Could you check a few things on this model? Use its own coordinates, in mm. Face numbers are marked on the shaded views. A direction names the side the tool comes from. Round coordinates to 2 decimals unless told otherwise and drop trailing zeros. Write each loop counter-clockwise with the first axis right and the second up, starting at its lowest first coordinate (ties: lowest second). Pieces come first, ordered by that corner, then holes. Notation, with made-up numbers: (21.5, -30) -> (79.5, -30) arc R11 cw to (79.5, -25) -> close; hole circle Ø8 at (10, 88.5). An arc over 180 degrees is marked (long way). Answer in a Markdown table with one row per item.
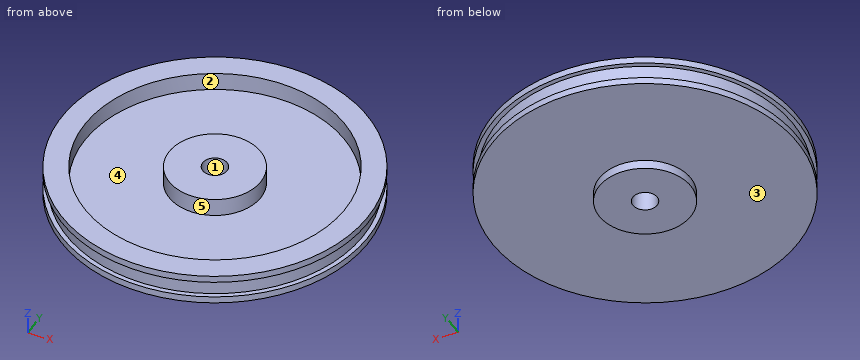
from build123d import *

# Parameters (mm, degrees)
SKETCH_1_R          = 100
EXTRUDE_1_DEPTH     = 20
SKETCH_2_R          = 8
CUT_EXTRUDE_1_DEPTH = 20
SKETCH_3_R          = 85
SKETCH_3_R_2        = 30
CUT_EXTRUDE_2_DEPTH = 12
SKETCH_5_W          = 3
SKETCH_5_H          = 11
SKETCH_8_R          = 30
EXTRUDE_2_DEPTH     = 6
CUT_EXTRUDE_START   = -52
SKETCH_9_R          = 8
CUT_EXTRUDE_4_DEPTH = 52


with BuildPart() as part:
    # 草图1 → 凸台-拉伸1 (new body)
    with BuildSketch(Plane.XY):
        Circle(SKETCH_1_R)
    extrude(amount=EXTRUDE_1_DEPTH)

    # 草图2 → 切除-拉伸1 (cut)
    with BuildSketch(Plane.XY.offset(20)):
        Circle(SKETCH_2_R)
    extrude(amount=-CUT_EXTRUDE_1_DEPTH, mode=Mode.SUBTRACT)

    # 草图3 → 切除-拉伸2 (cut)
    with BuildSketch(Plane.XY.offset(20)):
        Circle(SKETCH_3_R)
        Circle(SKETCH_3_R_2, mode=Mode.SUBTRACT)
    extrude(amount=-CUT_EXTRUDE_2_DEPTH, mode=Mode.SUBTRACT)

    # 草图5 → 切除-旋转2 (revolve, cut)
    with BuildSketch(Plane(origin=(0, 0, 0), x_dir=(1, 0, 0), z_dir=(0, 1, 0)), mode=Mode.PRIVATE) as cut_revolve_2_sk:
        with Locations((98.5, -10)):
            Rectangle(SKETCH_5_W, SKETCH_5_H)
    revolve(cut_revolve_2_sk.sketch.rotate(Axis((0, 0, -40.303548102), (0, 0, 1)), 180), axis=Axis((0, 0, -40.303548102), (0, 0, 1)), mode=Mode.SUBTRACT)

    # 草图8 → 凸台-拉伸2 (add)
    with BuildSketch(Plane(origin=(0, 0, 0), x_dir=(-1, 0, 0), z_dir=(0, 0, -1))):
        with Locations(Location((0, 0, 0), (0, 0, 180))):
            Circle(SKETCH_8_R)
    extrude(amount=EXTRUDE_2_DEPTH)

    # 草图9 → 切除-拉伸4 (cut)
    with BuildSketch(Plane(origin=(0, 0, -6), x_dir=(-1, 0, 0), z_dir=(0, 0, -1)).offset(CUT_EXTRUDE_START)):
        with Locations(Location((0, 0, 0), (0, 0, 180))):
            Circle(SKETCH_9_R)
    extrude(amount=CUT_EXTRUDE_4_DEPTH, mode=Mode.SUBTRACT)


solid = part.part
1) Imagine slicing it at C-C, the plane y = -50.5. Please give me the cut outline in (x, z).
Findings:
| item | result |
|---|---|
| outline | (-86.31, 0) -> (86.31, 0) -> (86.31, 4.5) -> (82.82, 4.5) -> (82.82, 15.5) -> (86.31, 15.5) -> (86.31, 20) -> (68.37, 20) -> (68.37, 8) -> (-68.37, 8) -> (-68.37, 20) -> (-86.31, 20) -> (-86.31, 15.5) -> (-82.82, 15.5) -> (-82.82, 4.5) -> (-86.31, 4.5) -> close |
2) For pin 1 (1 mm diameter, centred on x = 2, z = 3, fed in from -Y); pin 2 (2 mm diameter, centred on x = -9, z = 15.5, fed in from +Y); pin 3 (3 mm diameter, centred on x = 4.5, y = 63.5, fed in from -Z), each with a flat end and sliding along its axis, tell me the tip position at first contact or that it passes through.
Findings:
| item | result |
|---|---|
| pin 1 | stops at y = -99.99 |
| pin 2 | stops at y = 99.68 |
| pin 3 | stops at z = 0 |
3) Imagine slicing it at D-D, the plane x = -55. Please give me the cut outline in (y, z), plus the area to 3 significant figures.
Findings:
| item | result |
|---|---|
| outline | (-83.52, 0) -> (83.52, 0) -> (83.52, 4.5) -> (79.9, 4.5) -> (79.9, 15.5) -> (83.52, 15.5) -> (83.52, 20) -> (64.81, 20) -> (64.81, 8) -> (-64.81, 8) -> (-64.81, 20) -> (-83.52, 20) -> (-83.52, 15.5) -> (-79.9, 15.5) -> (-79.9, 4.5) -> (-83.52, 4.5) -> close |
| area | 1,710 mm^2 |
4) Please list where these lines run through material, in increasing order: line 1 (Y direction, x = 0, z = 14.5); line 2 (Y direction, x = 0, z = 2.25); line 3 (Y direction, x = -16, z = 12.5).
Findings:
| item | result |
|---|---|
| line 1 | y = -97 to -85, -30 to -8, 8 to 30, 85 to 97 |
| line 2 | y = -100 to -8, 8 to 100 |
| line 3 | y = -95.67 to -83.48, -25.38 to 25.38, 83.48 to 95.67 |
5) Imagine slicing it at A-A, the plane y = 0. Please give me the cut outline in (x, z), plus the area to 3 significant figures.
Findings:
| item | result |
|---|---|
| outline | (-100, 0) -> (-30, 0) -> (-30, -6) -> (-8, -6) -> (-8, 20) -> (-30, 20) -> (-30, 8) -> (-85, 8) -> (-85, 20) -> (-100, 20) -> (-100, 15.5) -> (-97, 15.5) -> (-97, 4.5) -> (-100, 4.5) -> close; (8, -6) -> (30, -6) -> (30, 0) -> (100, 0) -> (100, 4.5) -> (97, 4.5) -> (97, 15.5) -> (100, 15.5) -> (100, 20) -> (85, 20) -> (85, 8) -> (30, 8) -> (30, 20) -> (8, 20) -> close |
| area | 2,560 mm^2 |
6) Thinking about a two-plate mould opening in X: for the marked faces 3, 4 and 5, which applies, +X half, -X half, draft (parallel to the pull), parting line (faces both ways), or undercut?
Findings:
| item | result |
|---|---|
| face 3 | draft |
| face 4 | undercut |
| face 5 | undercut |
7) For the marked faces 1 and 2, which set-ups out of +Z, -Z, +X, -X, +Y, -Y let a thin tool reach every point of the face, with its end or its side?
Findings:
| item | result |
|---|---|
| face 1 | +Z, -Z |
| face 2 | +Z |
